Verification items for the finished model (mm, model axes). A direction names the side the tool comes from. Round coordinates to 2 decimals unless told otherwise and drop trailing zeros. Order: outer loops, then holes, each group sorted by start corner. A loop starts at its lowest first (then second) coordinate and runs counter-clockwise, first axis right, second up. Notation, with made-up numbers: (50.25, 85.25) -> (89.25, 85.25) arc R23 ccw to (89.25, 96.25) -> close; hole circle Ø3 at (-11, 23). An arc over 180 degrees is marked (long way). Return JSON: item names as keys, results as strings. Group by question number.
Item 1: Sectioned sample at A-A on x = -15. Record the cut outline in (y, z).
Item 2: Access from +Z, -Z, +X, -X, +Y, -Y to the whole of each face (thin tool, end or side, straight path). Record for faces 1 (the flat face through (7.645, 16.241, 0.986)), 2 (the flat face through (-2.3, 0.1, 0)).
Item 3: Depth check by flat-ended pin: pin 1 Ø1 at (y, z) = (-15, 0.5) entering from -X; pin 2 Ø1 at (x, z) = (5.5, 0.5) entering from -Y; pin 3 Ø0.6 at (x, z) = (-13.5, 1) entering from +Y. Enter the tip coordinate at first touch or a pass-through.
Item 4: Draft check along Y on faces 3 (the flat face through (-2.3, 0.1, 2)), 4 (the flat face through (9.744, -8.878, 1.014)). Enter one of: pulls with the +Y half, pulls with the -Y half, needs draft (parallel to the pull), parting line crosses it, or undercut.
Item 5: Sectioned sample at B-B on x = 5. Record the cut outline in (y, z), plus the area to 3 significant figures.
Item 6: Sectioned sample at C-C on x = 16.5. Record the cut outline in (y, z).
Item 7: Sectioned sample at D-D on z = 1. Give the number of separate pieces and of enclosed holes in the cut face, plus the area to 3 significant figures.
Item 8: Scan lines: probe 1 along Y at (x, z) = (0, 1.35); probe 2 along X at (y, z) = (6.5, 1.25); probe 3 along X at (y, z) = (-14.5, 0.45). Record each from-to range of solid material in increasing order. Write a range as from..to.
```python
from build123d import *

# Parameters (mm, degrees)
SKETCH_1_R          = 29
SKETCH_1_R_2        = 2
EXTRUDE_1_DEPTH     = 2
CUT_EXTRUDE_1_DEPTH = 2


with BuildPart() as part:
    # 草图1 → 凸台-拉伸1 (new body)
    with BuildSketch(Plane.XY):
        Circle(SKETCH_1_R)
        Circle(SKETCH_1_R_2, mode=Mode.SUBTRACT)
        with BuildLine():
            Line((-10, -1.5), (-26, -1.5))
            ThreePointArc((-26, -1.5), (-27.5, 0), (-26, 1.5))
            Line((-26, 1.5), (-10, 1.5))
            ThreePointArc((-10, 1.5), (-8.5, 0), (-10, -1.5))
        make_face(mode=Mode.SUBTRACT)
        with BuildLine():
            Line((3.700961894, 9.410254038), (11.700961894, 23.266660498))
            ThreePointArc((11.700961894, 23.266660498), (13.75, 23.815698604), (14.299038106, 21.766660498))
            Line((14.299038106, 21.766660498), (6.299038106, 7.910254038))
            ThreePointArc((6.299038106, 7.910254038), (4.25, 7.361215932), (3.700961894, 9.410254038))
        make_face(mode=Mode.SUBTRACT)
        with BuildLine():
            Line((6.299038106, -7.910254038), (14.299038106, -21.766660498))
            ThreePointArc((14.299038106, -21.766660498), (13.75, -23.815698604), (11.700961894, -23.266660498))
            Line((11.700961894, -23.266660498), (3.700961894, -9.410254038))
            ThreePointArc((3.700961894, -9.410254038), (4.25, -7.361215932), (6.299038106, -7.910254038))
        make_face(mode=Mode.SUBTRACT)
    extrude(amount=EXTRUDE_1_DEPTH)

    # 草图2 → 切除-拉伸1 (cut)
    with BuildSketch(Plane.XY.offset(2)):
        with BuildLine():
            Line((-18.973665961, 4), (-6.32455532, 4))
            ThreePointArc((-6.32455532, 4), (-4.816998597, 4.232687054), (-3.449757447, 4.909090909))
            ThreePointArc((-3.449757447, 4.909090909), (-3, 5.196152423), (-2.526518713, 5.442123041))
            ThreePointArc((-2.526518713, 5.442123041), (-1.257115216, 6.287986682), (-0.301823955, 7.477225575))
            Line((-0.301823955, 7.477225575), (6.022731365, 18.431676725))
            ThreePointArc((6.022731365, 18.431676725), (6.120040233, 23.254995789), (2.095605381, 25.915409279))
            ThreePointArc((2.095605381, 25.915409279), (-13, 22.516660498), (-23.491205476, 11.142857143))
            ThreePointArc((-23.491205476, 11.142857143), (-23.199437235, 6.327387581), (-18.973665961, 4))
        make_face()
        with BuildLine():
            Line((-18.973665961, -4), (-6.32455532, -4))
            ThreePointArc((-6.32455532, -4), (-4.816998597, -4.232687054), (-3.449757447, -4.909090909))
            ThreePointArc((-3.449757447, -4.909090909), (-3, -5.196152423), (-2.526518713, -5.442123041))
            ThreePointArc((-2.526518713, -5.442123041), (-1.257115216, -6.287986682), (-0.301823955, -7.477225575))
            Line((-0.301823955, -7.477225575), (6.022731365, -18.431676725))
            ThreePointArc((6.022731365, -18.431676725), (6.120040233, -23.254995789), (2.095605381, -25.915409279))
            ThreePointArc((2.095605381, -25.915409279), (-13, -22.516660498), (-23.491205476, -11.142857143))
            ThreePointArc((-23.491205476, -11.142857143), (-23.199437235, -6.327387581), (-18.973665961, -4))
        make_face()
        with BuildLine():
            Line((12.950934596, 14.431676725), (6.626379275, 3.477225575))
            ThreePointArc((6.626379275, 3.477225575), (6.074113814, 2.055299628), (5.97627616, 0.533032132))
            ThreePointArc((5.97627616, 0.533032132), (6, 0), (5.97627616, -0.533032132))
            ThreePointArc((5.97627616, -0.533032132), (6.074113814, -2.055299628), (6.626379275, -3.477225575))
            Line((6.626379275, -3.477225575), (12.950934596, -14.431676725))
            ThreePointArc((12.950934596, -14.431676725), (17.079397002, -16.927608208), (21.395600094, -14.772552136))
            ThreePointArc((21.395600094, -14.772552136), (26, 0), (21.395600094, 14.772552136))
            ThreePointArc((21.395600094, 14.772552136), (17.079397002, 16.927608208), (12.950934596, 14.431676725))
        make_face()
    extrude(amount=-CUT_EXTRUDE_1_DEPTH, mode=Mode.SUBTRACT)


solid = part.part
```
Recorded:
{
 "1": {"outline": "(-24.82, 0) -> (-21.24, 0) -> (-21.24, 2) -> (-24.82, 2) -> close; (-4, 0) -> (-1.5, 0) -> (-1.5, 2) -> (-4, 2) -> close; (1.5, 0) -> (4, 0) -> (4, 2) -> (1.5, 2) -> close; (21.24, 0) -> (24.82, 0) -> (24.82, 2) -> (21.24, 2) -> close"},
 "2": {"face 1": "+Z, -Z", "face 2": "-Z, +X, -X, +Y, -Y"},
 "3": {"pin 1": "x = -25.11", "pin 2": "y = -28.57", "pin 3": "y = 25.82"},
 "4": {"face 3": "needs draft", "face 4": "undercut"},
 "5": {"outline": "(-28.57, 0) -> (-24.68, 0) -> (-24.68, 2) -> (-28.57, 2) -> close; (-16.66, 0) -> (-11.66, 0) -> (-11.66, 2) -> (-16.66, 2) -> close; (-7.16, 0) -> (7.16, 0) -> (7.16, 2) -> (-7.16, 2) -> close; (11.66, 0) -> (16.66, 0) -> (16.66, 2) -> (11.66, 2) -> close; (24.68, 0) -> (28.57, 0) -> (28.57, 2) -> (24.68, 2) -> close", "area": "64.2 mm²"},
 "6": {"outline": "(-23.85, 0) -> (-16.87, 0) -> (-16.87, 2) -> (-23.85, 2) -> close; (16.87, 0) -> (23.85, 0) -> (23.85, 2) -> (16.87, 2) -> close"},
 "7": {"separate pieces": "1", "enclosed holes": "7", "area": "1,010 mm²"},
 "8": {"probe 1": "-29..-26, -8..-2, 2..8, 26..29", "probe 2": "-28.26..-23.3, -1.04..8.37, 25.17..28.26", "probe 3": "-25.11..-21.58, 3.75..6.64, 10.1..12.99, 21.58..25.11"}
}
